Here's the drawing with two shaded views (mm, measured from the low corner). I have some questions. Round coordinates to 2 decimals unless told otherwise and drop trailing zeros. Loops run counter-clockwise (first coordinate to the right, second up) from the corner with the lowest first, then second, coordinate; pieces in that order, holes last. Notation, with made-up numbers: (68.5, -26) -> (118.5, -26) arc R5 cw to (118.5, -19) -> close; hole circle Ø11 at (-11.5, 48.25). An arc over 180 degrees is marked (long way). Write item = value, one per line.
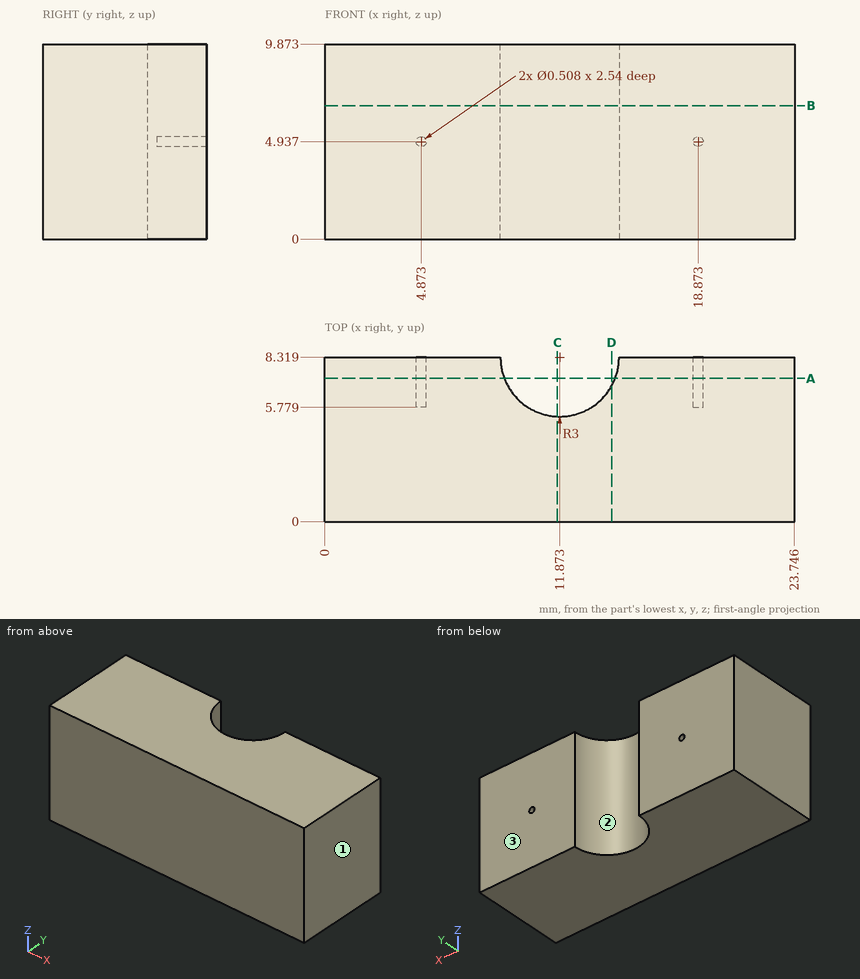
1. We'd pull the mould along X, two halves only. Please class the marked faces 1, 2 and 3: released by +X, released by -X, zero draft, split by the parting line, or undercut.
Entries:
face_1 = released by +X
face_2 = undercut
face_3 = zero draft
2. Suppose I cut it at A-A, the plane y = 7.25. List the corners of the cut face in (x, z) for me (1 decimal), and give its area (3 significant figures).
Entries:
outline = (0, 0) -> (9.1, 0) -> (9.1, 9.9) -> (0, 9.9) -> close; (14.7, 0) -> (23.7, 0) -> (23.7, 9.9) -> (14.7, 9.9) -> close; hole circle Ø0.5 at (4.9, 4.9); hole circle Ø0.5 at (18.9, 4.9)
area = 179 mm²
3. I need wall thicknesses on line 1 (X direction, y = 6.5, z = 4.75) (1 decimal); line 2 (X direction, y = 6, z = 8.5) (1 decimal); line 3 (X direction, y = 7.75, z = 2.5) (1 decimal). Which ranges of each line are inside material? Lowest first, please. Write a range as [from, to].
Entries:
line_1 = [0, 4.7], [5, 9.5], [14.3, 18.7], [19, 23.7]
line_2 = [0, 10], [13.8, 23.7]
line_3 = [0, 8.9], [14.8, 23.7]
4. Suppose I cut it at D-D, the plane x = 14.5. List the corners of the cut face in (y, z) for me.
Entries:
outline = (0, 0) -> (6.87, 0) -> (6.87, 9.87) -> (0, 9.87) -> close
5. Suppose I cut it at C-C, the plane x = 11.75. List the corners of the cut face in (y, z) for me.
Entries:
outline = (0, 0) -> (5.32, 0) -> (5.32, 9.87) -> (0, 9.87) -> close
6. Suppose I cut it at B-B, the plane z = 6.75. List the corners of the cut face in (x, y) for me (1 decimal), and give its area (3 significant figures).
Entries:
outline = (0, 0) -> (23.7, 0) -> (23.7, 8.3) -> (14.9, 8.3) arc R3 cw to (8.9, 8.3) -> (0, 8.3) -> close
area = 183 mm²
